from build123d import *

# Parameters (mm, degrees)
EXTRUDE_1_DEPTH     = 150
SKETCH_2_R          = 5
CUT_EXTRUDE_1_DEPTH = 33


with BuildPart() as part:
    # Эскиз1 → Вытянуть-Тонкостенный1 (new body)
    with BuildSketch(Plane(origin=(0, 0, 0), x_dir=(0, 0, -1), z_dir=(1, 0, 0))):
        Polygon((32, 0), (0, 0), (0, 32), (4, 32), (4, 4), (32, 4), align=None)
    extrude(amount=EXTRUDE_1_DEPTH)

    # Эскиз2 → Вырез-Вытянуть1 (cut, through all)
    with BuildSketch(Plane.XZ):
        with Locations((130, -13)):
            Circle(SKETCH_2_R)
        with Locations((100, -13)):
            Circle(SKETCH_2_R)
        with Locations((50, -13)):
            Circle(SKETCH_2_R)
        with Locations((20, -13)):
            Circle(SKETCH_2_R)
    extrude(amount=-CUT_EXTRUDE_1_DEPTH, mode=Mode.SUBTRACT)


solid = part.part
Read the model definition and answer for the solid it produces. Units are mm, in the model's axes. A direction names the side the tool comes from. Coordinates: 2 decimals unless noted, no trailing zeros. Order: outer loops, then holes, each group sorted by start corner. A loop starts at its lowest first (then second) coordinate and runs counter-clockwise, first axis right, second up. Notation, with made-up numbers: M 57,58 L 65,58 A17 cw 65,78 Z; hole C 63.5,86.25 d8. An arc over 180 degrees is marked long. Put each result on its own line as item: value. Start each with the question number.
Item 1: Section A-A, the plane x = 20 is taken. Determine the outline of the cut face in (y, z), plus the area to 3 significant figures.
Item 2: The mould has two halves that part along X. Classify faces 1 (the face through (150, 3, -9)), 2 (the face through (0, 3, -9)), 3 (the face through (24.77, 1.97, -11.5)), 4 (the face through (74, 4, -18)): +X half, -X half, draft (parallel to the pull), parting line (faces both ways), or undercut.
Item 3: Section C-C, the plane x = 88 is taken. Determine the outline of the cut face in (y, z), plus the area to 3 significant figures.
Item 4: For faces 5 (the face through (74, 18, -4)), 6 (the face through (74, 0, -16)), determine the directions among +Z, -Z, +X, -X, +Y, -Y from which every point of the face is accessible in a straight line to the end or side of a thin tool.
Item 5: Section D-D, the plane z = -28.5 is taken. Determine the outline of the cut face in (x, y), plus the area to 3 significant figures.
Item 6: Section B-B, the plane y = 29 is taken. Determine the outline of the cut face in (x, z).
Item 7: Consider probe 1 along Z at (x, y) = (50, 1); probe 2 along X at (y, z) = (2, -16); probe 3 along Z at (x, y) = (17, 9). Determine where each line is inside the solid, lowest interval first. Write a range as [from, to].
Item 8: Given pin 1 Ø10 at (x, z) = (112.5, -19) entering from +Y; pin 2 Ø10 at (x, y) = (81.5, 16.5) entering from -Z, each flat-ended and moving along its own axis, determine where each tip first touches the part or whether it passes through.
Computed:
1. outline: M 0,-32 L 4,-32 L 4,-18 L 0,-18 Z; M 0,-8 L 4,-8 L 4,-4 L 32,-4 L 32,0 L 0,0 Z
1. area: 200 mm2
2. face 1: +X half
2. face 2: -X half
2. face 3: undercut
2. face 4: draft
3. outline: M 0,-32 L 4,-32 L 4,-4 L 32,-4 L 32,0 L 0,0 Z
3. area: 240 mm2
4. face 5: -Z, +X, -X, +Y
4. face 6: +Z, -Z, +X, -X, -Y
5. outline: M 0,0 L 150,0 L 150,4 L 0,4 Z
5. area: 600 mm2
6. outline: M 0,-4 L 150,-4 L 150,0 L 0,0 Z
7. probe 1: z = [-32, -18], [-8, 0]
7. probe 2: x = [0, 16], [24, 46], [54, 96], [104, 126], [134, 150]
7. probe 3: z = [-4, 0]
8. pin 1: stops at y = 4
8. pin 2: stops at z = -4
